```python
from build123d import *

# Parameters (mm, degrees)
SKETCH1_R           = 24.13
SKETCH1_R_2         = 19.05
BOSS_EXTRUDE1_DEPTH = 6.35
SKETCH2_R           = 2.286
BOSS_EXTRUDE2_DEPTH = 2.54
SKETCH3_R           = 2.286
BOSS_EXTRUDE3_DEPTH = 2.54


with BuildPart() as part:
    # Sketch1 → Boss-Extrude1 (new body)
    with BuildSketch(Plane(origin=(0, 0, 0), x_dir=(1, 0, 0), z_dir=(0, 1, 0))):
        with Locations(Location((0, 0, 0), (0, 0, 270))):
            Circle(SKETCH1_R)
        with Locations(Location((0, 0, 0), (0, 0, 270))):
            Circle(SKETCH1_R_2, mode=Mode.SUBTRACT)
    extrude(amount=BOSS_EXTRUDE1_DEPTH)

    # Sketch2 → Boss-Extrude2 (add)
    with BuildSketch(Plane.XZ):
        with BuildLine():
            Line((21.809620202, 10.324600072), (21.809620202, -10.324600072))
            ThreePointArc((21.809620202, -10.324600072), (24.708155319, -6.688622381), (28.923046533, -4.724816982))
            ThreePointArc((28.923046533, -4.724816982), (32.766, 0), (28.923046533, 4.724816982))
            ThreePointArc((28.923046533, 4.724816982), (24.708155319, 6.688622381), (21.809620202, 10.324600072))
        make_face()
        with Locations(Location((27.94, 0, 0), (0, 0, 270))):
            Circle(SKETCH2_R, mode=Mode.SUBTRACT)
    extrude(amount=-BOSS_EXTRUDE2_DEPTH)

    # Sketch3 → Boss-Extrude3 (add)
    # profile 1 of 2: a face of its own
    with BuildSketch(Plane.XZ):
        with BuildLine():
            ThreePointArc((-18.110069721, 33.3113894), (-20.447664077, 33.59782849), (-22.371361767, 34.956424059))
            ThreePointArc((-22.371361767, 34.956424059), (-17.836458254, 24.069997968), (-20.578970769, 12.600113575))
            ThreePointArc((-20.578970769, 12.600113575), (-10.636194217, 21.659369164), (2.611644249, 23.988251589))
            ThreePointArc((2.611644249, 23.988251589), (-8.141414639, 28.83091072), (-13.983266974, 39.075537809))
            ThreePointArc((-13.983266974, 39.075537809), (-14.084369292, 36.722630449), (-15.286943189, 34.697732735))
            ThreePointArc((-15.286943189, 34.697732735), (-12.284263254, 29.563582193), (-7.99462004, 25.443564027))
            ThreePointArc((-7.99462004, 25.443564027), (-11.755793609, 23.93930276), (-15.245764429, 21.882768723))
            ThreePointArc((-15.245764429, 21.882768723), (-15.883236559, 27.796246369), (-18.110069721, 33.3113894))
        make_face()
    # profile 2 of 2: a face of its own
    with BuildSketch(Plane.XZ):
        with BuildLine():
            ThreePointArc((-22.371361767, 34.956424059), (-16.582401157, 33.768126167), (-13.983266974, 39.075537809))
            ThreePointArc((-13.983266974, 39.075537809), (-20.836878843, 42.431873833), (-22.371361767, 34.956424059))
        make_face()
        with Locations(Location((-18.70964, 38.1, 0), (0, 0, 270))):
            Circle(SKETCH3_R, mode=Mode.SUBTRACT)
    boss_extrude3 = extrude(amount=-BOSS_EXTRUDE3_DEPTH)

    # Mirror1: Boss-Extrude3 across plane
    add(boss_extrude3.mirror(Plane.XY))


solid = part.part
```
Verification items for the finished model (mm, model axes). Round coordinates to 2 decimals unless told otherwise and drop trailing zeros. Write each loop counter-clockwise with the first axis right and the second up, starting at its lowest first coordinate (ties: lowest second). Pieces come first, ordered by that corner, then holes.
1. Section check A-A on z = 0. Enter the section's corners in (x, y), plus the area to 3 significant figures.
2. Scan lines: L1, parallel to X at y = 1, z = 30.5; L2, parallel to X at y = 3.5, z = -13; L3, parallel to X at y = 2.5, z = -20. Record each from-to range of solid material in increasing order.
3. Draft check along X on faces 1 (the flat face through (26, 2.54, -1.5)), 2 (the cylindrical face through (-8.02, 1.25, 28.72)), 3 (the cylindrical face through (-15.863, 1.252, -27.715)). Enter one of: +X half, -X half, draft (parallel to the pull), parting line (faces both ways), or undercut.
4. Gauge pin test, flat ends, axial feed: P1, Ø3.5, axis at x = -18.71, z = 38.1, coming from the +Y side; P2, Ø2, axis at y = 4.5, z = 10.5, coming from the +X side; P3, Ø2, axis at x = -6.5, y = 4, coming from the +Z side. Record the tip position at first contact, or that the pin passes through.
5. Section check C-C on z = -38.1. Enter the section's corners in (x, y).
6. Section check B-B on x = 0. Enter the section's corners in (y, z).
7. Section check D-D on z = 17. Enter the section's corners in (x, y).
Answer:
1. outline: (-24.13, 0) - (-19.05, 0) - (-19.05, 6.35) - (-24.13, 6.35) - close; (19.05, 0) - (25.65, 0) - (25.65, 2.54) - (24.13, 2.54) - (24.13, 6.35) - (19.05, 6.35) - close; (30.23, 0) - (32.77, 0) - (32.77, 2.54) - (30.23, 2.54) - close
1. area: 74.8 mm2
2. L1: x = -19.51 to -16.75, -12.98 to -9.77
2. L2: x = -20.33 to -13.92, 13.92 to 20.33
2. L3: x = -17.95 to 13.5
3. face 1: draft
3. face 2: +X half
3. face 3: undercut
4. P1: passes through
4. P2: stops at x = 22.18
4. P3: stops at z = 23.49
5. outline: (-23.54, 0) - (-21, 0) - (-21, 2.54) - (-23.54, 2.54) - close; (-16.42, 0) - (-13.76, 0) - (-13.76, 2.54) - (-16.42, 2.54) - close
6. outline: (0, -24.46) - (2.54, -24.46) - (2.54, -24.13) - (6.35, -24.13) - (6.35, -19.05) - (0, -19.05) - close; (0, 19.05) - (6.35, 19.05) - (6.35, 24.13) - (2.54, 24.13) - (2.54, 24.46) - (0, 24.46) - close
7. outline: (-18.6, 0) - (-8.6, 0) - (-8.6, 6.35) - (-17.12, 6.35) - (-17.12, 2.54) - (-18.6, 2.54) - close; (8.6, 0) - (17.12, 0) - (17.12, 6.35) - (8.6, 6.35) - close
